Study the drawing (mm; zero at the part's minimum x, y, z) and answer. Give positions to 0.01 mm unless a question says otherwise; leave off trailing zeros. Order: outer loops, then holes, each group sorted by start corner. A loop starts at its lowest first (then second) coordinate and runs counter-clockwise, first axis right, second up.
Item 1: Find the intervals of material crossed by line 1 along X through (y, z) = (5, 29.6) (3 decimals); line 2 along Z through (x, y) = (141.7, 3.75) (3 decimals); line 3 along X through (y, z) = (2, 81), in increasing order.
Item 2: A cutting plane is placed at B-B (x = 5.9). Write down the section's boundary in (y, z) (3 decimals).
Item 3: A cutting plane is placed at A-A (z = 80.4). Write down the section's boundary in (x, y) (3 decimals).
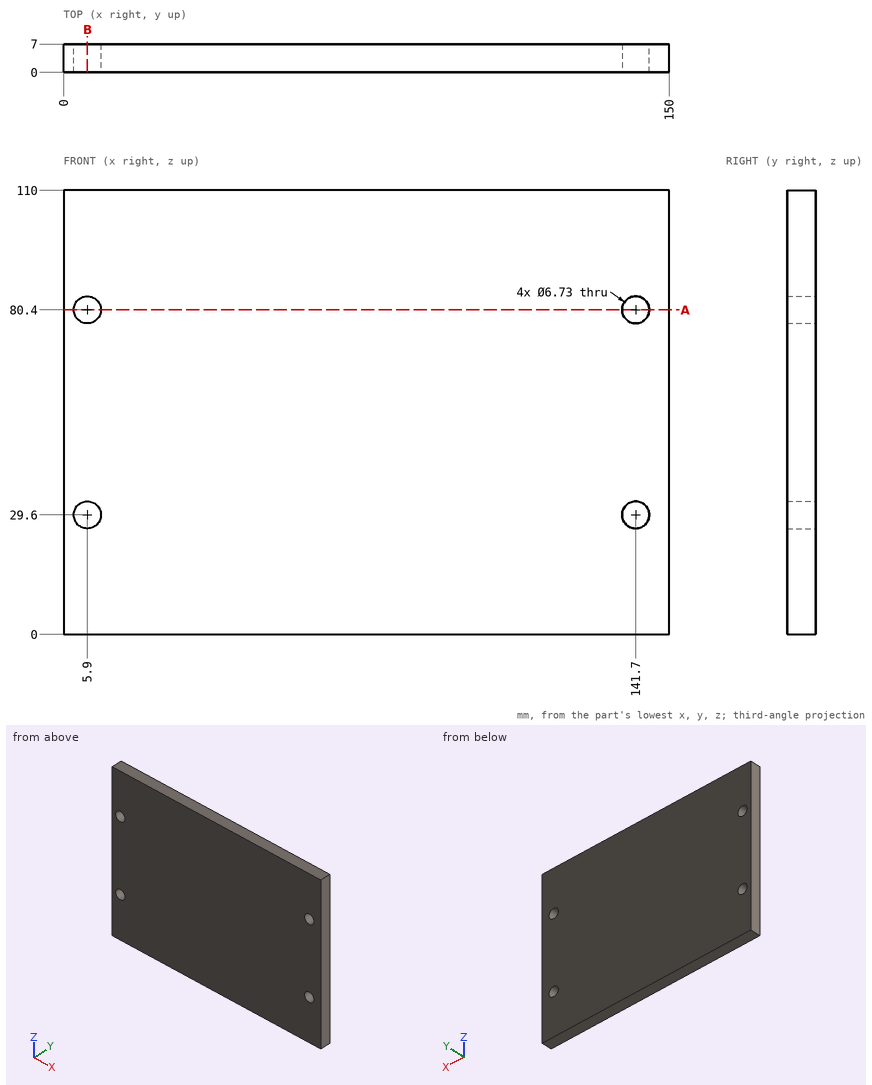
Response values:
1. line 1: x = 0 to 2.535, 9.265 to 138.335, 145.065 to 150
1. line 2: z = 0 to 26.235, 32.965 to 77.035, 83.765 to 110
1. line 3: x = 0 to 2.59, 9.21 to 138.39, 145.01 to 150
2. outline: (0, 0) - (7, 0) - (7, 26.235) - (0, 26.235) - close; (0, 32.965) - (7, 32.965) - (7, 77.035) - (0, 77.035) - close; (0, 83.765) - (7, 83.765) - (7, 110) - (0, 110) - close
3. outline: (0, 0) - (2.535, 0) - (2.535, 7) - (0, 7) - close; (9.265, 0) - (138.335, 0) - (138.335, 7) - (9.265, 7) - close; (145.065, 0) - (150, 0) - (150, 7) - (145.065, 7) - close
